```python
from build123d import *

# Parameters (mm, degrees)
SKETCH_1_W      = 95
SKETCH_1_H      = 40
SKETCH_1_R      = 2.5
EXTRUDE_1_DEPTH = 2


with BuildPart() as part:
    # 草图1 → 凸台-拉伸1 (new body)
    with BuildSketch(Plane.XY):
        with Locations((10, 0)):
            Rectangle(SKETCH_1_W, SKETCH_1_H)
        with Locations((7.5, 10)):
            Circle(SKETCH_1_R, mode=Mode.SUBTRACT)
        with Locations((12.5, -10)):
            Circle(SKETCH_1_R, mode=Mode.SUBTRACT)
        with Locations(Location((-29.5, -10, 0), (0, 0, 180))):
            Circle(SKETCH_1_R, mode=Mode.SUBTRACT)
        with Locations(Location((49.5, 10, 0), (0, 0, 180))):
            Circle(SKETCH_1_R, mode=Mode.SUBTRACT)
    extrude(amount=EXTRUDE_1_DEPTH)


solid = part.part
```
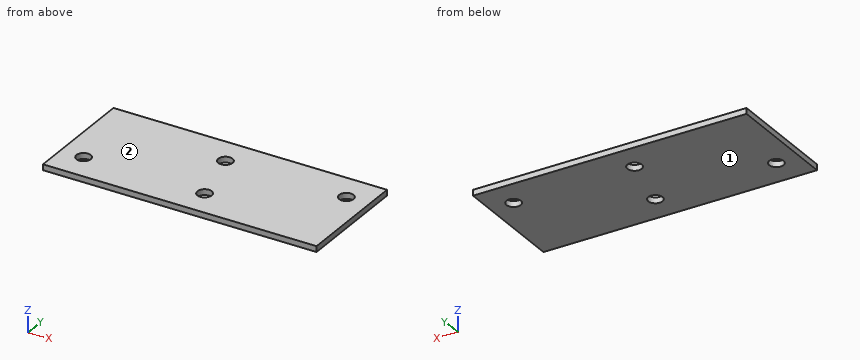
Source: CAD feature listing. Evaluate the final solid. Frame: model axes, mm. Face numbers are marked on the shaded views. Give positions to 0.01 mm unless a question says otherwise; leave off trailing zeros. Loops run counter-clockwise (first coordinate to the right, second up) from the corner with the lowest first, then second, coordinate; pieces in that order, holes last. Notation, with made-up numbers: (-12.75, -21) - (11.25, -21) arc R19 ccw to (11.25, 10) - close; hole circle Ø2 at (-21, -19). An arc over 180 degrees is marked (long way). Use CSV: the item, a comma, the result in double quotes. Start each with the question number.
1. Section B-B (y = -10). Output: boundary loops of the cut face in (x, z).
2. Section C-C (z = 0.8). Output: boundary loops of the cut face in (x, y), then the cut area to 3 significant figures.
3. Pin query (flat end, axial travel): pin 1 (3 mm diameter, centred on x = 49.5, y = 10, fed in from -Z). Return the tip coordinate at first contact, or that it passes through.
4. Draft query along Z for the marked faces 1 and 2. Return one class per face: +Z half, -Z half, draft (parallel to the pull), parting line (faces both ways), or undercut.
5. Section D-D (x = 11). Output: boundary loops of the cut face in (y, z), then the cut area to 3 significant figures.
6. Section A-A (x = 49.5). Output: boundary loops of the cut face in (y, z), then the cut area to 3 significant figures.
7. Ray query, L1, parallel to Y at x = -29.5, z = 1.15; L2, parallel to Y at x = 7.5, z = 0.9; L3, parallel to X at y = -8, z = 1.55. Return the intervals inside material, ascending.
Response:
1,outline,"(-37.5, 0) - (-32, 0) - (-32, 2) - (-37.5, 2) - close; (-27, 0) - (10, 0) - (10, 2) - (-27, 2) - close; (15, 0) - (57.5, 0) - (57.5, 2) - (15, 2) - close"
2,outline,"(-37.5, -20) - (57.5, -20) - (57.5, 20) - (-37.5, 20) - close; hole circle Ø5 at (-29.5, -10); hole circle Ø5 at (7.5, 10); hole circle Ø5 at (12.5, -10); hole circle Ø5 at (49.5, 10)"
2,area,"3,720 mm²"
3,pin 1,"through"
4,face 1,"-Z half"
4,face 2,"+Z half"
5,outline,"(-20, 0) - (-12, 0) - (-12, 2) - (-20, 2) - close; (-8, 0) - (20, 0) - (20, 2) - (-8, 2) - close"
5,area,"72.0 mm²"
6,outline,"(-20, 0) - (7.5, 0) - (7.5, 2) - (-20, 2) - close; (12.5, 0) - (20, 0) - (20, 2) - (12.5, 2) - close"
6,area,"70.0 mm²"
7,L1,"-20 to -12.5, -7.5 to 20"
7,L2,"-20 to 7.5, 12.5 to 20"
7,L3,"-37.5 to -31, -28 to 11, 14 to 57.5"
